Build history of the part. All positions in model axes, mm. Give positions to 0.01 mm unless a question says otherwise; leave off trailing zeros. Loops run counter-clockwise (first coordinate to the right, second up) from the corner with the lowest first, then second, coordinate; pieces in that order, holes last. Notation, with made-up numbers: (-16.5, 35.5) -> (9.5, 35.5) arc R26 ccw to (9.5, 66.5) -> close; hole circle Ø4 at (71, -32). An arc over 180 degrees is marked (long way). Answer as a JSON object with one key per item and string values. Group by question number.
Q1. Band-saw the part on D-D, the plane x = -7.75. Write the cut outline in (y, z).
Q2. Band-saw the part on C-C, the plane z = 0.2. Write the cut outline in (x, y).
Q3. Band-saw the part on A-A, the plane y = 0. Write the cut outline in (x, z).
Q4. Wall check: probe 1 along Y at (x, z) = (0, 0.3); probe 2 along Y at (x, z) = (-7.75, 0.4); probe 3 along Y at (x, z) = (-8.5, 0.2). Give the ranges that are in metal, low to high. Write a range as from..to.
Q5. Band-saw the part on B-B, the plane x = -3.5. Write the cut outline in (y, z), plus the area to 3 significant figures.
Q6. Drop a flat-ended pin along its axis: pin 1 (3 mm diameter, centred on x = -7.75, y = -13.42, fed in from +Z). Give the stop position or say it passes through.
from build123d import *

# Parameters (mm, degrees)
F0_R     = 19.5
F0_R_2   = 1.55
F0_R_3   = 6
F1_DEPTH = 1


with BuildPart() as f1:
    # F0 (on Top) → F1 (new body)
    with BuildSketch(Plane.XY):
        Circle(F0_R)
        with Locations((-7.75, -13.423394)):
            Circle(F0_R_2, mode=Mode.SUBTRACT)
        with Locations((-7.75, 13.423394)):
            Circle(F0_R_2, mode=Mode.SUBTRACT)
        with Locations((0, 7)):
            Circle(F0_R_3, mode=Mode.SUBTRACT)
        with Locations((15.5, 0)):
            Circle(F0_R_2, mode=Mode.SUBTRACT)
    extrude(amount=F1_DEPTH)


solid = f1.part
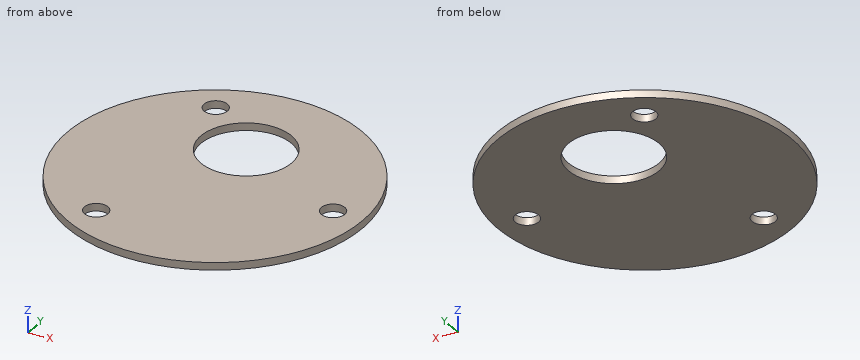
Worked answers:
{
 "1": {"outline": "(-17.89, 0) -> (-14.97, 0) -> (-14.97, 1) -> (-17.89, 1) -> close; (-11.87, 0) -> (11.87, 0) -> (11.87, 1) -> (-11.87, 1) -> close; (14.97, 0) -> (17.89, 0) -> (17.89, 1) -> (14.97, 1) -> close"},
 "2": {"outline": "circle Ø39 at (0, 0); hole circle Ø3.1 at (-7.75, -13.42); hole circle Ø3.1 at (-7.75, 13.42); hole circle Ø12 at (0, 7); hole circle Ø3.1 at (15.5, 0)"},
 "3": {"outline": "(-19.5, 0) -> (13.95, 0) -> (13.95, 1) -> (-19.5, 1) -> close; (17.05, 0) -> (19.5, 0) -> (19.5, 1) -> (17.05, 1) -> close"},
 "4": {"probe 1": "-19.5..1, 13..19.5", "probe 2": "-17.89..-14.97, -11.87..11.87, 14.97..17.89", "probe 3": "-17.55..-14.78, -12.07..12.07, 14.78..17.55"},
 "5": {"outline": "(-19.18, 0) -> (2.13, 0) -> (2.13, 1) -> (-19.18, 1) -> close; (11.87, 0) -> (19.18, 0) -> (19.18, 1) -> (11.87, 1) -> close", "area": "28.6 mm2"},
 "6": {"pin 1": "through"}
}
